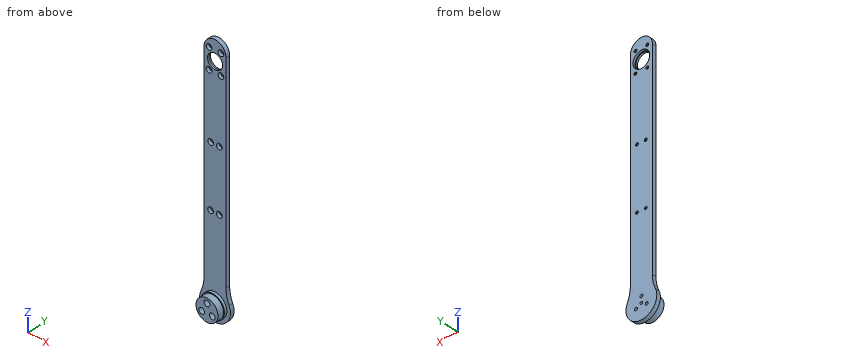
```python
from build123d import *
from build123d.topology import SkipClean

# Parameters (mm, degrees)
EXTRUDE_1_DEPTH              = 9
SKETCH_3_R                   = 13.5
EXTRUDE_2_DEPTH              = 2
SKETCH_4_R                   = 13.5
EXTRUDE_3_DEPTH              = 3
SKETCH_5_R                   = 9.5
CUT_EXTRUDE_2_DEPTH          = 274.324898244
HOLE_WIZARD_M3_4_D           = 3.4
HOLE_WIZARD_M3_4_CBORE_D     = 6.5
HOLE_WIZARD_M3_4_CBORE_DEPTH = 3.4
PATTERN_CIRCULAR_1_COUNT     = 3
SKETCH_11_R                  = 12.5
SKETCH_11_R_2                = 3.25
EXTRUDE_4_DEPTH              = 7
SKETCH_13_R                  = 11
CUT_EXTRUDE_3_DEPTH          = 3
FILLET_1_R                   = 40
SKETCH_26_W                  = 65.136073631
SKETCH_26_H                  = 16.815092821
CUT_EXTRUDE_5_DEPTH          = 1111
SKETCH_28_R                  = 9.5
SKETCH_28_R_2                = 8.5
EXTRUDE_5_DEPTH              = 2
HOLE_WIZARD_M3_2_D           = 3.2
HOLE_WIZARD_M3_2_CBORE_D     = 6.5
HOLE_WIZARD_M3_2_CBORE_DEPTH = 3.4
PATTERN_LINEAR_1_COUNT       = 3
PATTERN_LINEAR_1_PITCH       = 70
PATTERN_LINEAR_1_COUNT_DIR2  = 2
PATTERN_LINEAR_1_PITCH_DIR2  = 10
HOLE_WIZARD_M3_3_D           = 3.2
HOLE_WIZARD_M3_3_CBORE_D     = 6.5
HOLE_WIZARD_M3_3_CBORE_DEPTH = 3.4
PATTERN_CIRCULAR_2_COUNT     = 6
SKETCH_39_R                  = 3.25
EXTRUDE_6_DEPTH              = 4.5
F_3_0MM_1_D                  = 3
F_3_0MM_1_DEPTH              = 5
F_3_0MM_1_TIP                = 0.901290929


with BuildPart() as part:
    # Sketch 1 → Extrude 1 (new body)
    with BuildSketch(Plane(origin=(0, 0, 0), x_dir=(1, 0, 0), z_dir=(0, 1, 0))):
        with BuildLine():
            Line((-12.5, -260), (-12.5, -12.247448714))
            ThreePointArc((-12.5, -12.247448714), (0, 17.5), (12.5, -12.247448714))
            Line((12.5, -12.247448714), (12.5, -260))
            ThreePointArc((12.5, -260), (0, -272.5), (-12.5, -260))
        make_face()
    extrude(amount=EXTRUDE_1_DEPTH)

    # Sketch 3 → Extrude 2 (add)
    with BuildSketch(Plane(origin=(0, 9, 0), x_dir=(1, 0, 0), z_dir=(0, 1, 0))):
        with Locations(Location((0, 0, 0), (0, 0, 270))):
            Circle(SKETCH_3_R)
    extrude(amount=EXTRUDE_2_DEPTH)

    # Sketch 4 → Extrude 3 (add)
    with BuildSketch(Plane.XZ):
        with Locations(Location((0, 0, 0), (0, 0, 90))):
            Circle(SKETCH_4_R)
    extrude(amount=EXTRUDE_3_DEPTH)

    # Sketch 5 → Cut-Extrude 2 (cut, through all)
    with BuildSketch(Plane(origin=(0, 9, 0), x_dir=(1, 0, 0), z_dir=(0, 1, 0))):
        with Locations(Location((0, -250, 0), (0, 0, 270))):
            Circle(SKETCH_5_R)
    extrude(amount=-CUT_EXTRUDE_2_DEPTH, mode=Mode.SUBTRACT)

    # Hole Wizard M3 _ _ _ _ _ _4 (through all)
    with Locations(Plane(origin=(0, -3, 0), x_dir=(-1, 0, 0), z_dir=(0, -1, 0))):
        with Locations((0, -7)):
            hole_wizard_m3_4 = CounterBoreHole(HOLE_WIZARD_M3_4_D / 2, HOLE_WIZARD_M3_4_CBORE_D / 2, HOLE_WIZARD_M3_4_CBORE_DEPTH)

    # Pattern Circular 1: Hole Wizard M3 _ _ _ _ _ _4 ×3 about axis
    pattern_circular_1_axis = Axis((0, 0, 0), (0, 1, 0))
    for i in range(1, PATTERN_CIRCULAR_1_COUNT):
        add(hole_wizard_m3_4.rotate(pattern_circular_1_axis, i * 360 / PATTERN_CIRCULAR_1_COUNT), mode=Mode.SUBTRACT)

    # Sketch 11 → Extrude 4 (add)
    with SkipClean():  # the faces are left unmerged after this step: merging them gives an invalid solid
        with BuildSketch(Plane.XZ.offset(3)):
            with Locations(Location((0, 0, 0), (0, 0, 270))):
                Circle(SKETCH_11_R)
            with Locations(Location((6.062177826, -3.5, 0), (0, 0, 270))):
                Circle(SKETCH_11_R_2, mode=Mode.SUBTRACT)
            with Locations(Location((0, 7, 0), (0, 0, 270))):
                Circle(SKETCH_11_R_2, mode=Mode.SUBTRACT)
            with Locations(Location((-6.062177826, -3.5, 0), (0, 0, 270))):
                Circle(SKETCH_11_R_2, mode=Mode.SUBTRACT)
        extrude(amount=EXTRUDE_4_DEPTH)

    # Sketch 13 → Cut-Extrude 3 (cut)
    with SkipClean():  # the faces are left unmerged after this step: merging them gives an invalid solid
        with BuildSketch(Plane(origin=(0, 11, 0), x_dir=(1, 0, 0), z_dir=(0, 1, 0))):
            with Locations(Location((0, 0, 0), (0, 0, 270))):
                Circle(SKETCH_13_R)
        extrude(amount=-CUT_EXTRUDE_3_DEPTH, mode=Mode.SUBTRACT)

    # Fillet 1
    fillet_1_edges = [part.edges().sort_by_distance(p)[0] for p in [
        (12.5, 4.5, 12.247448714),
        (-12.5, 4.5, 12.247448714),
    ]]
    fillet(fillet_1_edges, radius=FILLET_1_R)

    # Sketch 26 → Cut-Extrude 5 (cut, symmetric)
    with BuildSketch(Plane.XY):
        with Locations((0.11753139, 12.907546411)):
            Rectangle(SKETCH_26_W, SKETCH_26_H)
    extrude(amount=CUT_EXTRUDE_5_DEPTH, both=True, mode=Mode.SUBTRACT)

    # Sketch 28 → Extrude 5 (add)
    with BuildSketch(Plane.XZ):
        with Locations(Location((0, 250, 0), (0, 0, 270))):
            Circle(SKETCH_28_R)
        with Locations(Location((0, 250, 0), (0, 0, 270))):
            Circle(SKETCH_28_R_2, mode=Mode.SUBTRACT)
    extrude(amount=-EXTRUDE_5_DEPTH)

    # Hole Wizard M3 _ _ _ _ _ _2 (through all)
    with Locations(Plane(origin=(0, 0, 0), x_dir=(-1, 0, 0), z_dir=(0, -1, 0))):
        with Locations((5, -25)):
            hole_wizard_m3_2 = CounterBoreHole(HOLE_WIZARD_M3_2_D / 2, HOLE_WIZARD_M3_2_CBORE_D / 2, HOLE_WIZARD_M3_2_CBORE_DEPTH)

    # Pattern Linear 1: Hole Wizard M3 _ _ _ _ _ _2 3 × 2
    with Locations(*[(j * PATTERN_LINEAR_1_PITCH_DIR2, 0, i * PATTERN_LINEAR_1_PITCH) for i in range(PATTERN_LINEAR_1_COUNT) for j in range(PATTERN_LINEAR_1_COUNT_DIR2) if (i, j) != (0, 0)]):
        add(hole_wizard_m3_2, mode=Mode.SUBTRACT)

    # Hole Wizard M3 _ _ _ _ _ _3 (through all)
    with Locations(Plane(origin=(0, 0, 0), x_dir=(-1, 0, 0), z_dir=(0, -1, 0))):
        with Locations((6.75, -261.691342951)):
            hole_wizard_m3_3 = CounterBoreHole(HOLE_WIZARD_M3_3_D / 2, HOLE_WIZARD_M3_3_CBORE_D / 2, HOLE_WIZARD_M3_3_CBORE_DEPTH)

    # Pattern Circular 2: Hole Wizard M3 _ _ _ _ _ _3 ×6 about axis, 2 skipped
    pattern_circular_2_axis = Axis((0, 2, 250), (0, -1, 0))
    add([hole_wizard_m3_3.rotate(pattern_circular_2_axis, i * 360 / PATTERN_CIRCULAR_2_COUNT) for i in range(1, PATTERN_CIRCULAR_2_COUNT) if i not in (1, 4)], mode=Mode.SUBTRACT)

    # Sketch 39 → Extrude 6 (add)
    with BuildSketch(Plane.XZ):
        with Locations((5, 25)):
            Circle(SKETCH_39_R)
        with Locations((-5, 25)):
            Circle(SKETCH_39_R)
    extrude(amount=-EXTRUDE_6_DEPTH)

    # 3.0mm _ _1
    with Locations(Plane(origin=(0, 4.5, 0), x_dir=(1, 0, 0), z_dir=(0, 1, 0))):
        with Locations((0, 0)):
            Hole(F_3_0MM_1_D / 2, depth=F_3_0MM_1_DEPTH)
            with Locations((0, 0, -(F_3_0MM_1_DEPTH + F_3_0MM_1_TIP / 2))):  # 118° drill point
                Cone(0, F_3_0MM_1_D / 2, F_3_0MM_1_TIP, mode=Mode.SUBTRACT)


solid = part.part
```
Build history of the part. All positions in model axes, mm. Give positions to 0.01 mm unless a question says otherwise; leave off trailing zeros. Order: outer loops, then holes, each group sorted by start corner. A loop starts at its lowest first (then second) coordinate and runs counter-clockwise, first axis right, second up. Notation, with made-up numbers: M 49,3 L 99,3 A28 cw 99,37 Z; hole C -26,-29.75 d11. An arc over 180 degrees is marked long. Return JSON: item names as keys, results as strings.
Q1. Wall check: probe 1 along X at (y, z) = (3.75, 95); probe 2 along X at (y, z) = (0.9, 165); probe 3 along Z at (x, y) = (6.75, 4.1). Give the ranges that are in metal, low to high. Write a range as from..to.
Answer list:
{"probe 1": "x = -12.5..-6.6, -3.4..3.4, 6.6..12.5", "probe 2": "x = -12.5..-8.25, -1.75..1.75, 8.25..12.5", "probe 3": "z = -16.15..-5.05, -1.95..236.71, 239.91..243.32, 256.68..260.09, 263.29..270.52"}
Q2. Band-saw the part on B-B (z = 182). Give the cut face in (x, y).
Answer list:
{"outline": "M -12.5,0 L 12.5,0 L 12.5,4.5 L -12.5,4.5 Z"}
Q3. Flat gauge pins, fed straight in: pin 1 (2.5 mm diameter, centred on y = 1.5, z = 120, fed in from -X); pin 2 (1.5 mm diameter, centred on y = -1, z = 106.5, fed in from +X); pin 3 (4 mm diameter, centred on x = 6.75, z = 238.31, fed in from -Y); pin 4 (6 mm diameter, centred on x = 11, z = 120, fed in from -Y). Where does each tip first touch, or does it go through?
Answer list:
{"pin 1": "stops at x = -12.5", "pin 2": "passes through", "pin 3": "stops at y = 3.4", "pin 4": "stops at y = 0"}
Q4. Band-saw the part on A-A (z = 250). Give the cut face in (x, y), then the cut area to 3 significant figures.
Answer list:
{"outline": "M -12.5,0 L -8.5,0 L -8.5,2 L -9.5,2 L -9.5,4.5 L -12.5,4.5 Z; M 8.5,0 L 12.5,0 L 12.5,4.5 L 9.5,4.5 L 9.5,2 L 8.5,2 Z", "area": "31.0 mm^2"}
